The listing builds one solid part. Answer for the finished solid, in the listing's coordinates (mm). A direction names the side the tool comes from. Coordinates: 2 decimals unless noted, no trailing zeros. Order: outer loops, then holes, each group sorted by start corner. A loop starts at its lowest first (then second) coordinate and runs counter-clockwise, first axis right, second up. Notation, with made-up numbers: (2, -24) -> (45, -24) arc R28 ccw to (45, -6) -> close; hole circle Ø5 at (29.25, 75.5). An arc over 180 degrees is marked (long way). Answer in a Markdown table with one row per item. Add a question column.
```python
from build123d import *

# Parameters (mm, degrees)
SKETCH_R  = 9.5
PAD_DEPTH = 10


with BuildPart() as part:
    # Sketch → Pad (new body)
    with BuildSketch(Plane.XY):
        Circle(SKETCH_R)
        with BuildLine():
            ThreePointArc((-3.75, 4.85), (-5.164214, 4.264214), (-5.75, 2.85))
            add(Edge.make_bspline(
                [(-5.75, 2.85), (-5.797957, 0.992558), (-5.136857, 1.384321), (-5.149992, -0.009195)],
                knots=[0, 0, 0, 0, 1, 1, 1, 1], degree=3))
            ThreePointArc((-5.149992, -0.009195), (0, -5.15), (5.149992, -0.009195))
            add(Edge.make_bspline(
                [(5.75, 2.85), (5.797957, 0.992558), (5.136857, 1.384321), (5.149992, -0.009195)],
                knots=[0, 0, 0, 0, 1, 1, 1, 1], degree=3))
            ThreePointArc((5.75, 2.85), (5.164214, 4.264214), (3.75, 4.85))
            Line((3.75, 4.85), (-3.75, 4.85))
        make_face(mode=Mode.SUBTRACT)
    extrude(amount=PAD_DEPTH)


solid = part.part
```
Q1. For faces 1 (the face through (4, -4, 0)), 2 (the face through (0, 4.85, 5)), determine the directions among +Z, -Z, +X, -X, +Y, -Y from which every point of the face is accessible in a straight line to the end or side of a thin tool.
Q2. A cutting plane is placed at A-A (x = 0). Determine the outline of the cut face in (y, z), then the cut area to 3 significant figures.
Q3. A cutting plane is placed at C-C (y = -5.5). Determine the outline of the cut face in (x, z).
Q4. A cutting plane is placed at D-D (y = 7.5). Determine the outline of the cut face in (x, z).
Q5. Straight lines are drawn through the part: line 1 (Y direction, x = 0.25, z = 6.75); line 2 (X direction, y = 4.25, z = 1); line 3 (X direction, y = 1.5, z = 2.25). For each, find the intervals that lie inside material, in ascending order.
Q6. A cutting plane is placed at B-B (y = -3.5). Determine the outline of the cut face in (x, z).
Q7. Determine the mould class of faces 3 (the face through (-5.15, 4.28, 4.93)), 4 (the face through (4, -4, 10)), 5 (the face through (4.38, -8.43, 4.93)) for opening direction Y: +Y half, -Y half, draft (parallel to the pull), parting line (faces both ways), or undercut.
Q8. Given pin 1 (2 mm diameter, centred on x = -6, z = 9, fed in from +Y); pin 2 (2 mm diameter, centred on x = 4, z = 3, fed in from +Y); pin 3 (6 mm diameter, centred on x = 0.5, y = -1, fed in from -Z); pin 4 (1 mm diameter, centred on y = -2.5, z = 6, fed in from -X), each flat-ended and moving along its own axis, determine where each tip first touches the part or whether it passes through.
Returned:
| question | item | result |
|---|---|---|
| 1 | face 1 | -Z, +X, -X, +Y, -Y |
| 1 | face 2 | +Z, -Z |
| 2 | outline | (-9.5, 0) -> (-5.15, 0) -> (-5.15, 10) -> (-9.5, 10) -> close; (4.85, 0) -> (9.5, 0) -> (9.5, 10) -> (4.85, 10) -> close |
| 2 | area | 90.0 mm² |
| 3 | outline | (-7.75, 0) -> (7.75, 0) -> (7.75, 10) -> (-7.75, 10) -> close |
| 4 | outline | (-5.83, 0) -> (5.83, 0) -> (5.83, 10) -> (-5.83, 10) -> close |
| 5 | line 1 | y = -9.5 to -5.14, 4.85 to 9.5 |
| 5 | line 2 | x = -8.5 to -5.18, 5.18 to 8.5 |
| 5 | line 3 | x = -9.38 to -5.58, 5.58 to 9.38 |
| 6 | outline | (-8.83, 0) -> (-3.78, 0) -> (-3.78, 10) -> (-8.83, 10) -> close; (3.78, 0) -> (8.83, 0) -> (8.83, 10) -> (3.78, 10) -> close |
| 7 | face 3 | undercut |
| 7 | face 4 | draft |
| 7 | face 5 | parting line |
| 8 | pin 1 | stops at y = 8.08 |
| 8 | pin 2 | stops at y = 9.01 |
| 8 | pin 3 | passes through |
| 8 | pin 4 | stops at x = -9.29 |
